The listing builds one solid part. Answer for the finished solid, in the listing's coordinates (mm). A direction names the side the tool comes from. Give positions to 0.01 mm unless a question says otherwise; leave off trailing zeros. Write each loop counter-clockwise with the first axis right and the second up, starting at its lowest first coordinate (ties: lowest second). Pieces come first, ordered by that corner, then holes. Notation, with made-up numbers: (-28, 70.5) -> (6, 70.5) arc R31 ccw to (6, 103.5) -> close; hole circle Ø10 at (36.5, 29.25). An arc over 180 degrees is marked (long way). One line per question, with ' | ' between items.
from build123d import *

# Parameters (mm, degrees)
F0_W      = 66.5
F0_H      = 80.5
F1_DEPTH  = 27
F2_T      = -2.5
F3_R      = 2
F4_W      = 49.75
F4_H      = 24.5
F5_DEPTH  = 25
F6_W      = 45.5
F6_H      = 48.5
F7_DEPTH  = 25
F8_W      = 48
F8_H      = 17.5
F9_DEPTH  = 25
F10_W     = 11.5
F10_H     = 26
F11_DEPTH = 25
F12_W     = 9
F12_H     = 14
F13_DEPTH = 25


with BuildPart() as f1:
    # F0 (on Front) → F1 (new body)
    with BuildSketch(Plane.XZ):
        with Locations((30.75, 37.75)):
            Rectangle(F0_W, F0_H)
    extrude(amount=F1_DEPTH)

    # F2
    f2_openings = [f1.faces().sort_by_distance(p)[0] for p in [
        (30.75, -27, 37.75),
    ]]
    offset(amount=F2_T, openings=f2_openings)

    # F3
    f3_edges = [f1.edges().sort_by_distance(p)[0] for p in [
        (64, -13.5, 78),
        (-2.5, -13.5, 78),
        (64, -13.5, -2.5),
        (-2.5, -13.5, -2.5),
    ]]
    fillet(f3_edges, radius=F3_R)

    # F4 (on face) → F5 (cut)
    with BuildSketch(Plane.XY):
        with Locations((34.125, -14.75)):
            Rectangle(F4_W, F4_H)
    extrude(amount=-F5_DEPTH, mode=Mode.SUBTRACT)

    # F6 (on face) → F7 (cut)
    with BuildSketch(Plane.XZ.offset(2.5)):
        with Locations((31.75, 41.25)):
            Rectangle(F6_W, F6_H)
    extrude(amount=-F7_DEPTH, mode=Mode.SUBTRACT)

    # F8 (on face) → F9 (cut)
    with BuildSketch(Plane(origin=(0, 0, 0), x_dir=(-1, 0, 0), z_dir=(0, 1, 0))):
        with Locations((-33, 6.25)):
            Rectangle(F8_W, F8_H)
    extrude(amount=-F9_DEPTH, mode=Mode.SUBTRACT)

    # F10 (on face) → F11 (cut)
    with BuildSketch(Plane(origin=(-2.5, 0, 0), x_dir=(0, -1, 0), z_dir=(-1, 0, 0))):
        with Locations((8.25, 15)):
            Rectangle(F10_W, F10_H)
    extrude(amount=-F11_DEPTH, mode=Mode.SUBTRACT)

    # F12 (on face) → F13 (cut)
    with BuildSketch(Plane.XZ.offset(2.5)):
        with Locations((4.5, 24)):
            Rectangle(F12_W, F12_H)
    extrude(amount=-F13_DEPTH, mode=Mode.SUBTRACT)


solid = f1.part
Item 1: A tool of negligible diameter and unlimited length cuts with its end or side. For faces 4 (the face through (57, -1, 6)), 5 (the face through (31, -1, 65.5)), 6 (the face through (5, -15, 0)), from which of +Z, -Z, +X, -X, +Y, -Y can it reach the whole face along a straight path? Write none if from no direction.
Answers below:
face 4: -Z, +Y, -Y | face 5: +Y, -Y | face 6: -Y
Item 2: Flat-ended cylindrical pins translate along their axes: pin 1 (7.5 mm diameter, centred on x = 28.5, y = -16.5, fed in from -Z); pin 2 (4 mm diameter, centred on x = 54, z = 8, fed in from -Y). Find the tip coordinate at first contact, or state that the pin passes through.
Answers below:
pin 1: z = 75.5 | pin 2: through
Item 3: Find section A-A (z = 48). Write down the section's boundary in (x, y).
Answers below:
outline: (-2.5, -27) -> (0, -27) -> (0, -2.5) -> (9, -2.5) -> (9, 0) -> (-2.5, 0) -> close; (54.5, -2.5) -> (61.5, -2.5) -> (61.5, -27) -> (64, -27) -> (64, 0) -> (54.5, 0) -> close
Item 4: Determine the mould class of faces 1 (the face through (-1, -8, 2)), 2 (the face through (26, 0, 68)), 3 (the face through (64, -13, 37)) for opening direction Y: pulls with the +Y half, pulls with the -Y half, needs draft (parallel to the pull), parting line crosses it, or undercut.
Answers below:
face 1: undercut | face 2: pulls with the +Y half | face 3: needs draft
Item 5: Find section B-B (y = -9.25). Write down the section's boundary in (x, z), then the cut area to 3 significant figures.
Answers below:
outline: (-2.5, -0.5) arc R2 ccw to (-0.5, -2.5) -> (9, -2.5) -> (9, 0) -> (0, 0) -> (0, 2) -> (-2.5, 2) -> close; (-2.5, 28) -> (0, 28) -> (0, 75.5) -> (61.5, 75.5) -> (61.5, 0) -> (59, 0) -> (59, -2.5) -> (62, -2.5) arc R2 ccw to (64, -0.5) -> (64, 76) arc R2 ccw to (62, 78) -> (-0.5, 78) arc R2 ccw to (-2.5, 76) -> close | area: 517 mm²
Item 6: Consider line 1 (X direction, y = -9.5, z = 68.5); line 2 (Z direction, x = 1.5, y = -9); line 3 (X direction, y = -1.5, z = 3). Determine where each line is inside the solid, lowest interval first. Write a range as [from, to].
Answers below:
line 1: [-2.5, 0], [61.5, 64] | line 2: [-2.5, 0], [75.5, 78] | line 3: [-2.5, 9], [57, 64]
Item 7: Find section D-D (z = 11.5). Write down the section's boundary in (x, y), then the cut area to 3 significant figures.
Answers below:
outline: (-2.5, -27) -> (0, -27) -> (0, -14) -> (-2.5, -14) -> close; (-2.5, -2.5) -> (9, -2.5) -> (9, 0) -> (-2.5, 0) -> close; (57, -2.5) -> (61.5, -2.5) -> (61.5, -27) -> (64, -27) -> (64, 0) -> (57, 0) -> close | area: 140 mm²
Item 8: Find section C-C (x = 11). Write down the section's boundary in (y, z).
Answers below:
outline: (-27, 75.5) -> (-2.5, 75.5) -> (-2.5, 65.5) -> (0, 65.5) -> (0, 78) -> (-27, 78) -> close; (-2.5, 15) -> (0, 15) -> (0, 17) -> (-2.5, 17) -> close
